Verification items for the finished model (mm, model axes). Give positions to 0.01 mm unless a question says otherwise; leave off trailing zeros. Order: outer loops, then holes, each group sorted by start corner. A loop starts at its lowest first (then second) coordinate and runs counter-clockwise, first axis right, second up. Notation, with made-up numbers: M 48,73 L 95,73 A32 ccw 95,100 Z; hole C -19,67.5 d1. An arc over 180 degrees is marked long. Answer as a JSON object with one key per item and string values.
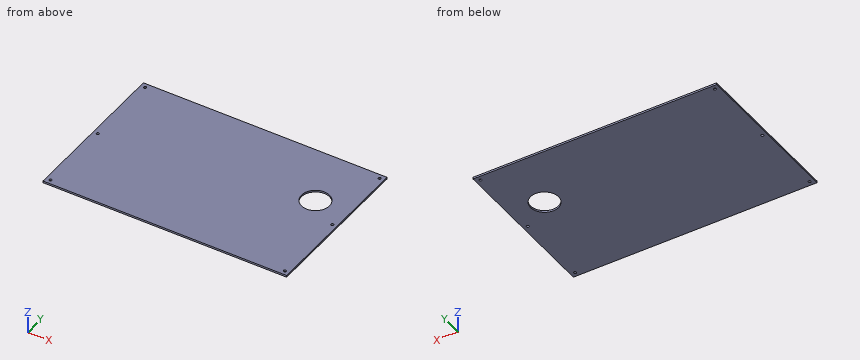
```python
from build123d import *

# Parameters (mm, degrees)
SKICA1_W                 = 535
SKICA1_H                 = 350
SKICA1_R                 = 3
P_IDAT_VYSUNUT_M1_DEPTH  = 4
SKICA2_R                 = 30.776653742
ODEBRAT_VYSUNUT_M1_DEPTH = 4


with BuildPart() as part:
    # Skica1 → Přidat vysunutím1 (new body)
    with BuildSketch(Plane.XY):
        Rectangle(SKICA1_W, SKICA1_H)
        with Locations((-257.5, 165)):
            Circle(SKICA1_R, mode=Mode.SUBTRACT)
        with Locations((-257.5, 0)):
            Circle(SKICA1_R, mode=Mode.SUBTRACT)
        with Locations((-257.5, -165)):
            Circle(SKICA1_R, mode=Mode.SUBTRACT)
        with Locations((257.5, 165)):
            Circle(SKICA1_R, mode=Mode.SUBTRACT)
        with Locations((257.5, 0)):
            Circle(SKICA1_R, mode=Mode.SUBTRACT)
        with Locations((257.5, -165)):
            Circle(SKICA1_R, mode=Mode.SUBTRACT)
    extrude(amount=P_IDAT_VYSUNUT_M1_DEPTH)

    # Skica2 → Odebrat vysunutím1 (cut)
    with BuildSketch(Plane(origin=(0, 0, 0), x_dir=(-1, 0, 0), z_dir=(0, 0, -1))):
        with Locations((-192.248320425, 45.04602447)):
            Circle(SKICA2_R)
    extrude(amount=-ODEBRAT_VYSUNUT_M1_DEPTH, mode=Mode.SUBTRACT)


solid = part.part
```
Q1. Gauge pin test, flat end, axial feed: pin 1 Ø5.5 at (x, y) = (-257.5, 0) entering from +Z. Record the tip position at first contact, or that the pin passes through.
Resolved:
{"pin 1": "passes through"}
Q2. Section check A-A on z = 1.65. Record the cut outline in (x, y), then the cut area to 3 significant figures.
Resolved:
{"outline": "M -267.5,-175 L 267.5,-175 L 267.5,175 L -267.5,175 Z; hole C -257.5,-165 d6; hole C -257.5,0 d6; hole C -257.5,165 d6; hole C 192.25,45.05 d61.55; hole C 257.5,-165 d6; hole C 257.5,0 d6; hole C 257.5,165 d6", "area": "184,000 mm²"}
Q3. Material ranges on L1, parallel to X at y = -165, z = 2.2; L2, parallel to Y at x = -257.5, z = 1.7; L3, parallel to X at y = 2.5, z = 2.15, recorded low to high.
Resolved:
{"L1": "x = -267.5 to -260.5, -254.5 to 254.5, 260.5 to 267.5", "L2": "y = -175 to -168, -162 to -3, 3 to 162, 168 to 175", "L3": "x = -267.5 to -259.16, -255.84 to 255.84, 259.16 to 267.5"}
